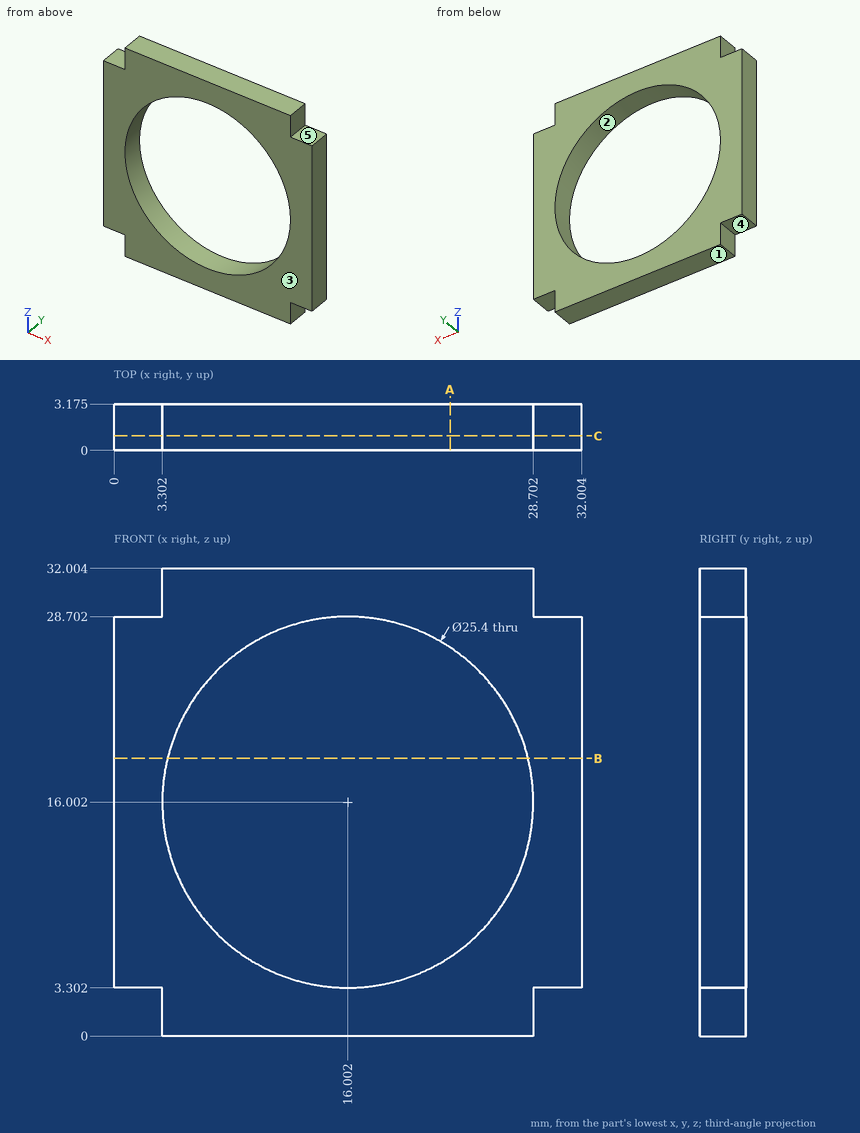
The figure shows three views and two pictorial views of one solid part (mm, origin at its lowest corner). Answer the questions. A direction names the side the tool comes from. Coordinates: 2 decimals unless noted, no trailing zeros. Loops run counter-clockwise (first coordinate to the right, second up) from the corner with the lowest first, then second, coordinate; pieces in that order, holes last. Notation, with made-up numbers: (64.25, 10) - (86.25, 10) arc R6 cw to (86.25, 19) - close; hole circle Ø9 at (-18, 42.25). An arc over 180 degrees is marked (long way). Use a Markdown table: item, result. Add a question column.
1) Given pin 1 (1 mm diameter, centred on y = 1.5, z = 1, fed in from +X); pin 2 (1 mm diameter, centred on x = 30, y = 1.5, fed in from -Z); pin 3 (1 mm diameter, centred on y = 1.5, z = 30.5, fed in from -X), each flat-ended and moving along its own axis, determine where each tip first touches the part or whether it passes through.
2) The part is cut by section B-B, the plane z = 19. Give the vertices of the cut face in (x, y) (3 decimals), and give its area (3 significant figures).
3) The mould has two halves that part along X. Classify the marked faces 1 and 2: released by +X, released by -X, zero draft, split by the parting line, or undercut.
4) The part is cut by section C-C, the plane y = 1. Give the vertices of the cut face in (x, z), and give its area (3 significant figures).
5) The part is cut by section A-A, the plane x = 23. Give the vertices of the cut face in (y, z) (3 decimals).
6) For the marked faces 3, 4 and 5, determine the directions among +Z, -Z, +X, -X, +Y, -Y from which every point of the face is accessible in a straight line to the end or side of a thin tool.
7) Find the intervals of material crossed by line 1 (X direction, y = 2.6, z = 29.5); line 2 (X direction, y = 1.05, z = 23); line 3 (X direction, y = 1, z = 10), in increasing order.
Here are the results:
| question | item | result |
|---|---|---|
| 1 | pin 1 | stops at x = 28.7 |
| 1 | pin 2 | stops at z = 3.3 |
| 1 | pin 3 | stops at x = 3.3 |
| 2 | outline | (0, 0) - (3.661, 0) - (3.661, 3.175) - (0, 3.175) - close; (28.343, 0) - (32.004, 0) - (32.004, 3.175) - (28.343, 3.175) - close |
| 2 | area | 23.2 mm^2 |
| 3 | face 1 | zero draft |
| 3 | face 2 | undercut |
| 4 | outline | (0, 3.3) - (3.3, 3.3) - (3.3, 0) - (28.7, 0) - (28.7, 3.3) - (32, 3.3) - (32, 28.7) - (28.7, 28.7) - (28.7, 32) - (3.3, 32) - (3.3, 28.7) - (0, 28.7) - close; hole circle Ø25.4 at (16, 16) |
| 4 | area | 474 mm^2 |
| 5 | outline | (0, 0) - (3.175, 0) - (3.175, 5.404) - (0, 5.404) - close; (0, 26.6) - (3.175, 26.6) - (3.175, 32.004) - (0, 32.004) - close |
| 6 | face 3 | +Z, -Z, +X, -X, -Y |
| 6 | face 4 | -Z, -X, +Y, -Y |
| 6 | face 5 | +Z, +X, +Y, -Y |
| 7 | line 1 | x = 3.3 to 28.7 |
| 7 | line 2 | x = 0 to 5.4, 26.6 to 32 |
| 7 | line 3 | x = 0 to 4.81, 27.19 to 32 |
